Verification items for this drawing (mm, ordinates from the low corner). A direction names the side the tool comes from. Coordinates: 2 decimals unless noted, no trailing zeros. Loops run counter-clockwise (first coordinate to the right, second up) from the corner with the lowest first, then second, coordinate; pieces in that order, holes last. Notation, with made-up numbers: (44, 43) - (64, 43) arc R11 ccw to (64, 55) - close; hole circle Ø6 at (14, 49.5). An arc over 180 degrees is marked (long way). One line per item, written item: value. Start each with the question number.
(1) Set-up check for the marked faces 1 and 2: record each of +Z, -Z, +X, -X, +Y, -Y from which the full face is reachable in a straight line by a thin tool's end or side.
(2) Draft check along Z on the marked faces 3 and 4. Enter one of: +Z half, -Z half, draft (parallel to the pull), parting line (faces both ways), or undercut.
(3) Thickness scan on probe 1 along X at (y, z) = (1.3, 62.5) (1 decimal); probe 2 along X at (y, z) = (1.25, 73); probe 3 along Z at (x, y) = (87, 1.95) (1 decimal). Record the ranges inside material, lowest first. Write a range as [from, to].
(4) Section check D-D (x = 91.5). Record the boundary of the cut face in (y, z) (1 decimal), plus the area to 3 significant figures.
(5) Section check C-C (z = 88.5). Record the boundary of the cut face in (x, y).
(6) Section check A-A (x = 50.5). Record the boundary of the cut face in (y, z) (1 decimal).
(7) Gauge pin test, flat end, axial feed: P1, Ø1, axis at y = 2, z = 44.5, coming from the +X side. Record the tip position at first contact, or that the pin passes through.
(8) Section check B-B (y = 0.4). Record the boundary of the cut face in (x, z), plus the area to 3 significant figures.
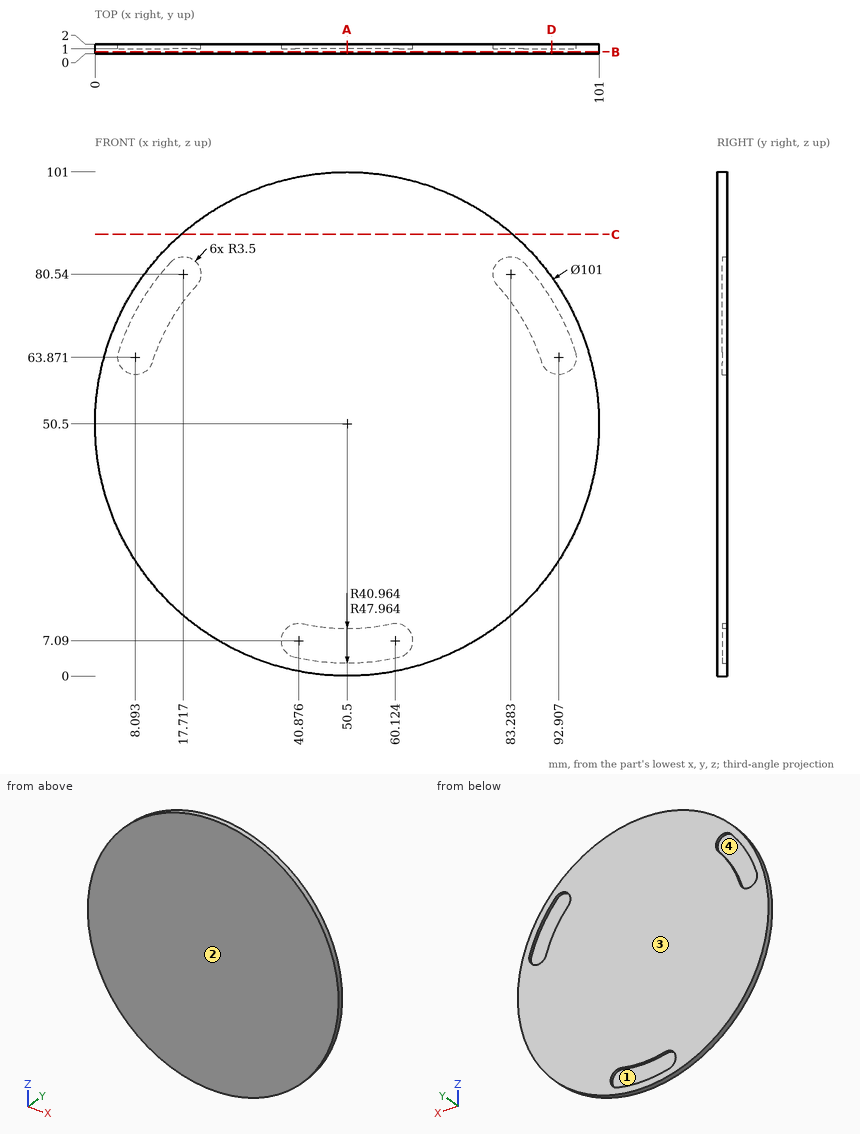
Responses:
1. face 1: +Y
1. face 2: +Z, -Z, +X, -X, -Y
2. face 3: draft
2. face 4: undercut
3. probe 1: x = [1.4, 4.9], [11.3, 89.7], [96.1, 99.6]
3. probe 2: x = [5.29, 8.14], [16.27, 84.73], [92.86, 95.71]
3. probe 3: z = [15.6, 69.1], [81.6, 85.4]
4. outline: (0, 21) - (2, 21) - (2, 60.7) - (1, 60.7) - (1, 75.4) - (2, 75.4) - (2, 80) - (0, 80) - close
4. area: 103 mm²
5. outline: (17.24, 0) - (83.76, 0) - (83.76, 2) - (17.24, 2) - close
6. outline: (0, 0) - (2, 0) - (2, 2.5) - (1, 2.5) - (1, 9.5) - (2, 9.5) - (2, 101) - (0, 101) - close
7. P1: stops at x = 100.7
8. outline: circle Ø101 at (50.5, 50.5)
8. area: 8,010 mm²
